Autodesk Inventor part; units mm, degrees
ref_plane "YZ Plane" through (0, 0, 0) normal (1, 0, 0) x (0, 1, 0)
ref_plane "XZ Plane" through (0, 0, 0) normal (0, 1, 0) x (-1, 0, 0)
ref_plane "XY Plane" through (0, 0, 0) normal (0, 0, 1) x (1, 0, 0)
sketch "Sketch1" plane through (0, 0, 0) normal (0, 0, 1) x (1, 0, 0)
  line L0 (0, 0) -> (25.3902, 0)
  line L1 (25.3902, 0) -> (25.3902, 3.175)
  line L2 (3.175, 50.8) -> (0, 50.8)
  line L3 (0, 50.8) -> (0, 0)
  line L4 (3.175, 50.8) -> (3.175, 3.175)
  line L5 (3.175, 3.175) -> (25.3902, 3.175)
  dimension "d0" = 50.8
  dimension "d1" = 25.3902
  dimension "d2" = 3.175
  dimension "d3" = 3.175
extrude "Extrusion1" add sketch "Sketch1" along normal blind 381
sketch "Sketch2" plane through (0, 0, 0) normal (0, -1, 0) x (1, 0, 0)
  line L0 (0, 0) -> (25.3902, 0)
  line L1 (25.3902, 0) -> (25.3902, 381)
  line L2 (25.3902, 158.75) -> (12.6902, 171.45)
  line L3 (12.6902, 171.45) -> (12.6902, 209.55)
  line L4 (12.6902, 209.55) -> (25.3902, 222.25)
  dimension "d6" = 12.7
  dimension "d7" = 45
  dimension "d8" = 45
  dimension "d9" = 38.1
  dimension "d10" = 171.45
extrude "Extrusion2" cut sketch "Sketch2" against normal through all
sketch "Sketch3" plane through (0, 0, 0) normal (-1, 0, 0) x (0, 0, 1)
  line L0 (381, 0) -> (381, 50.8)
  line L1 (0, 50.8) -> (381, 50.8)
  line L2 (0, 50.8) -> (0, 0)
  line L3 (0, 0) -> (381, 0)
  line L4 (50.8, 50.8) -> (76.2, 25.4)
  line L5 (76.2, 25.4) -> (304.8, 25.4)
  line L6 (304.8, 25.4) -> (330.2, 50.8)
  dimension "d13" = 25.4
  dimension "d14" = 45
  dimension "d15" = 45
  dimension "d16" = 50.8
  dimension "d17" = 50.8
extrude "Extrusion3" cut sketch "Sketch3" against normal through all contours L6 L5 L4 L1
equation "\"d2\" = d3"
equation "\"d7\" = d8"
equation "\"d15\" = d14"
equation "\"d17\" = d16"
properties part number "8 ball  frame bottom L"
Input: part model. Units: mm. Frame: model coordinates. A direction names the side the tool comes from. Give positions to 0.01 mm unless a question says otherwise; leave off trailing zeros. Order: outer loops, then holes, each group sorted by start corner. A loop starts at its lowest first (then second) coordinate and runs counter-clockwise, first axis right, second up.
Q1. Section B-B on x = 20.25. Output: boundary loops of the cut face in (y, z) (3 decimals).
Checked values:
outline: (0, 0) - (3.175, 0) - (3.175, 163.89) - (0, 163.89) - close; (0, 217.11) - (3.175, 217.11) - (3.175, 381) - (0, 381) - close
Q2. Contact query for flat-ended pins moving along their axis: pin 1 Ø3.5 at (y, z) = (1.5, 182) entering from +X; pin 2 Ø2.5 at (x, z) = (1, 229) entering from +Y; pin 3 Ø1.5 at (x, z) = (12.5, 194.5) entering from +Y (3 decimals). Output: stop coordinate, or through.
Checked values:
pin 1: stops at x = 12.69
pin 2: stops at y = 25.4
pin 3: stops at y = 3.175
Q3. Ray query, probe 1 along X at (y, z) = (35.5, 354) (3 decimals); probe 2 along X at (y, z) = (3, 185). Return the intervals inside material, ascending.
Checked values:
probe 1: x = 0 to 3.175
probe 2: x = 0 to 12.69
Q4. Section D-D on y = 18.5. Output: boundary loops of the cut face in (x, z) (3 decimals).
Checked values:
outline: (0, 0) - (3.175, 0) - (3.175, 381) - (0, 381) - close
Q5. Section A-A on y = 41. Output: boundary loops of the cut face in (x, z) (3 decimals).
Checked values:
outline: (0, 0) - (3.175, 0) - (3.175, 60.6) - (0, 60.6) - close; (0, 320.4) - (3.175, 320.4) - (3.175, 381) - (0, 381) - close
Q6. Draft query along Z for faces 6 (the flat face through (1.6, 37.9, 317.3)), 7 (the flat face through (2, 18, 381)), 8 (the flat face through (12.5, 0, 187.8)). Return one class per face: +Z half, -Z half, draft (parallel to the pull), parting line (faces both ways), or undercut.
Checked values:
face 6: undercut
face 7: +Z half
face 8: draft
Q7. Section C-C on z = 234. Output: boundary loops of the cut face in (x, y) (3 decimals), and give its area (3 significant figures).
Checked values:
outline: (0, 0) - (25.39, 0) - (25.39, 3.175) - (3.175, 3.175) - (3.175, 25.4) - (0, 25.4) - close
area: 151 mm2
Q8. Set-up query: faces 1 (the flat face through (18.95, 1.57, 215.81)), 2 (the flat face through (0, 20, 188)), 3 (the flat face through (12, 3.175, 188)), 4 (the flat face through (2, 18, 0)), 5 (the flat face through (1.6, 38.3, 63.3)). Return all of +Z, -Z, +X, -X, +Y, -Y with unobstructed straight access to the full face (end or side cutting, diameter ignored); none if empty.
Checked values:
face 1: +X, +Y, -Y
face 2: +Z, -Z, -X, +Y, -Y
face 3: +Z, -Z, +X, +Y
face 4: -Z, +X, -X, +Y, -Y
face 5: +X, -X, +Y
